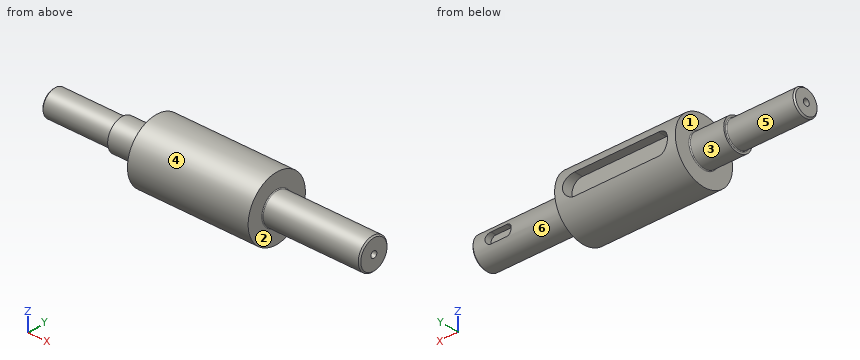
```python
from build123d import *

# Parameters (mm, degrees)
CUT_EXTRUDE1_START              = 8
CUT_EXTRUDE1_DEPTH              = 4
SKETCH3_W                       = 8
SKETCH3_H                       = 5
CUT_EXTRUDE2_DEPTH              = 10
SKETCH4_R                       = 1.25
CUT_EXTRUDE3_DEPTH              = 4
SKETCH5_R                       = 6
CUT_EXTRUDE4_DEPTH              = 10
CUT_EXTRUDE5_START              = 6
CUT_EXTRUDE5_DEPTH              = 2.5
M3_TAPPED_HOLE1_D               = 2.5
M3_TAPPED_HOLE1_DEPTH           = 6.748924226
M3_TAPPED_HOLE1_TIP             = 0.751075774
M3_TAPPED_HOLE1_ON_FACE_2_D     = 2.5
M3_TAPPED_HOLE1_ON_FACE_2_DEPTH = 6.748924226
M3_TAPPED_HOLE1_ON_FACE_2_TIP   = 0.751075774
CHAMFER1_SIZE                   = 0.5
FILLET1_R                       = 0.3


with BuildPart() as part:
    # Sketch1 → Revolve1 (revolve)
    with BuildSketch(Plane.XY):
        Polygon((26, 6), (60, 6), (70, 6), (70, 0), (60, 0), (-60, 0), (-62, 0), (-62, 5), (-36, 5), (-36, 6), (-23, 6), (-23, 12), (23, 12), (23, 6), align=None)
    revolve(axis=Axis((60, 0, 0), (-1, 0, 0)))

    # Sketch2 → Cut-Extrude1 (cut)
    with BuildSketch(Plane(origin=(0, 0, 0), x_dir=(1, 0, 0), z_dir=(0, 1, 0)).offset(CUT_EXTRUDE1_START)):
        with BuildLine():
            Line((-16, 4), (16, 4))
            ThreePointArc((16, 4), (20, 0), (16, -4))
            Line((16, -4), (-16, -4))
            ThreePointArc((-16, -4), (-20, 0), (-16, 4))
        make_face()
    extrude(amount=CUT_EXTRUDE1_DEPTH, mode=Mode.SUBTRACT)

    # Sketch3 → Cut-Extrude2 (cut)
    with BuildSketch(Plane(origin=(70, 0, 0), x_dir=(0, 0, -1), z_dir=(1, 0, 0))):
        with Locations((0, 7)):
            Rectangle(SKETCH3_W, SKETCH3_H)
    extrude(amount=-CUT_EXTRUDE2_DEPTH, mode=Mode.SUBTRACT)

    # Sketch4 → Cut-Extrude3 (cut)
    with BuildSketch(Plane(origin=(0, 4.5, 0), x_dir=(1, 0, 0), z_dir=(0, 1, 0))):
        with Locations((65, 0)):
            Circle(SKETCH4_R)
    extrude(amount=-CUT_EXTRUDE3_DEPTH, mode=Mode.SUBTRACT)

    # Sketch5 → Cut-Extrude4 (cut)
    with BuildSketch(Plane(origin=(60, 0, 0), x_dir=(0, 0, -1), z_dir=(1, 0, 0))):
        Circle(SKETCH5_R)
    extrude(amount=CUT_EXTRUDE4_DEPTH, mode=Mode.SUBTRACT)

    # Sketch7 → Cut-Extrude5 (cut)
    with BuildSketch(Plane(origin=(0, 0, 0), x_dir=(1, 0, 0), z_dir=(0, 1, 0)).offset(CUT_EXTRUDE5_START)):
        with BuildLine():
            Line((47, 2), (53, 2))
            ThreePointArc((53, 2), (55, 0), (53, -2))
            Line((53, -2), (47, -2))
            ThreePointArc((47, -2), (45, 0), (47, 2))
        make_face()
    extrude(amount=-CUT_EXTRUDE5_DEPTH, mode=Mode.SUBTRACT)

    # M3 Tapped Hole1
    with Locations(Plane(origin=(-62, 0, 0), x_dir=(0, -1, 0), z_dir=(-1, 0, 0))):
        with Locations((0, 0)):
            Hole(M3_TAPPED_HOLE1_D / 2, depth=M3_TAPPED_HOLE1_DEPTH)
            with Locations((0, 0, -(M3_TAPPED_HOLE1_DEPTH + M3_TAPPED_HOLE1_TIP / 2))):  # 118° drill point
                Cone(0, M3_TAPPED_HOLE1_D / 2, M3_TAPPED_HOLE1_TIP, mode=Mode.SUBTRACT)

    # M3 Tapped Hole1 on face 2
    with Locations(Plane(origin=(60, 0, 0), x_dir=(0, 0, 1), z_dir=(1, 0, 0))):
        with Locations((0, 0)):
            Hole(M3_TAPPED_HOLE1_ON_FACE_2_D / 2, depth=M3_TAPPED_HOLE1_ON_FACE_2_DEPTH)
            with Locations((0, 0, -(M3_TAPPED_HOLE1_ON_FACE_2_DEPTH + M3_TAPPED_HOLE1_ON_FACE_2_TIP / 2))):  # 118° drill point
                Cone(0, M3_TAPPED_HOLE1_ON_FACE_2_D / 2, M3_TAPPED_HOLE1_ON_FACE_2_TIP, mode=Mode.SUBTRACT)

    # Chamfer1
    chamfer1_edges = [part.edges().sort_by_distance(p)[0] for p in [
        (-62, -5, 0),
        (60, -6, 0),
    ]]
    chamfer(chamfer1_edges, length=CHAMFER1_SIZE)

    # Fillet1
    fillet1_edges = [part.edges().sort_by_distance(p)[0] for p in [
        (-36, -5, 0),
        (-23, -6, 0),
        (23, -6, 0),
    ]]
    fillet(fillet1_edges, radius=FILLET1_R)


solid = part.part
```
Design review of the part built by this model. Coordinates are the model's own, in mm. Face numbers are marked on the shaded views. A direction names the side the tool comes from. Round coordinates to 2 decimals unless told otherwise and drop trailing zeros. Order: outer loops, then holes, each group sorted by start corner. A loop starts at its lowest first (then second) coordinate and runs counter-clockwise, first axis right, second up. Notation, with made-up numbers: M -21,-3 L 5,-3 A22 ccw 5,13 Z; hole C -9.75,61.25 d9. An arc over 180 degrees is marked long. Put each result on its own line as item: value.
Q1. Machinability: for the marked faces 4, 5 and 6, which of the approach directions +Z, -Z, +X, -X, +Y, -Y give a long, thin tool a straight path to every point of the face, cutting with its end or side? Answer none if there is none.
Reported:
face 4: +X, -X
face 5: -X
face 6: +X
Q2. Consider section D-D (z = 7.75). State the section outline as (x, y) points.
Reported:
outline: M -23,-9.16 L 23,-9.16 L 23,9.16 L -23,9.16 Z
Q3. Consider section A-A (y = 9.25). State the section outline as (x, z) points.
Reported:
outline: M -23,-7.64 L 23,-7.64 L 23,7.64 L -23,7.64 Z; hole M -16,-4 L 16,-4 A4 ccw 16,4 L -16,4 A4 ccw Z
Q4. To check wall thickness, follow line 1 (Z direction, x = -59.25, y = 0); line 2 (Y direction, x = 55.25, z = 0); line 3 (X direction, y = 4, z = 5.25). State the ranges of each line that lie inside material, in increasing order.
Reported:
line 1: -5 to -1.25, 1.25 to 5
line 2: -6 to -1.25, 1.25 to 6
line 3: -23 to 23
Q5. Consider section C-C (y = -8). State the section outline as (x, z) points, and give its area (3 significant figures).
Reported:
outline: M -23,-8.94 L 23,-8.94 L 23,8.94 L -23,8.94 Z
area: 823 mm²
Q6. Consider section B-B (x = 43). State the section outline as (y, z) points, and give its area (3 significant figures).
Reported:
outline: C 0,0 d12
area: 113 mm²
Q7. Draft analysis for pull direction X (two halves, no side actions). For the marked faces 1, 2 and 3, state which applies: released by +X, released by -X, zero draft, split by the parting line, or undercut.
Reported:
face 1: released by -X
face 2: released by +X
face 3: zero draft
Q8. Insertion check: pin 1 Ø6.5 at (x, z) = (6, 0) entering from +Y; pin 2 Ø1.5 at (y, z) = (0, -8.5) entering from -X; pin 3 Ø2.5 at (x, y) = (49.5, 4) entering from +Z; pin 4 Ø3 at (x, y) = (-29.5, 8) entering from +Z. Each pin has a flat end and moves straight along its axis. Give the tip position at first contact, or say it passes through.
Reported:
pin 1: y = 8
pin 2: x = -23
pin 3: z = 5.33
pin 4: through
